Read the model definition and answer for the solid it produces. Units are mm, in the model's axes. Coordinates: 2 decimals unless noted, no trailing zeros. Loops run counter-clockwise (first coordinate to the right, second up) from the corner with the lowest first, then second, coordinate; pieces in that order, holes last. Notation, with made-up numbers: (35, 75) - (79, 75) arc R22 ccw to (79, 104) - close; hole circle Ø9 at (47, 0.25). An arc over 180 degrees is marked (long way). Use one line per item in the form item = value. Start each with the question number.
1) A cutting plane is placed at B-B (y = -42). Give the vertices of the cut face in (x, z), and give its area (3 significant figures).
2) Each of these flat-tipped pins is pushed along its axis until it touches: P1, Ø5, axis at x = 71.51, y = -164.45, coming from the +Z side; P2, Ø0.9, axis at x = 37, z = -2.5, coming from the +Y side. Where does it stop, or does it pass through?
3) Consider line 1 (X direction, y = -184, z = -2.6); line 2 (X direction, y = -74.45, z = -1.95); line 3 (Y direction, x = 67, z = -1.8). Determine where each line is inside the solid, lowest interval first.
4) A cutting plane is placed at A-A (y = -184). Give the vertices of the cut face in (x, z).
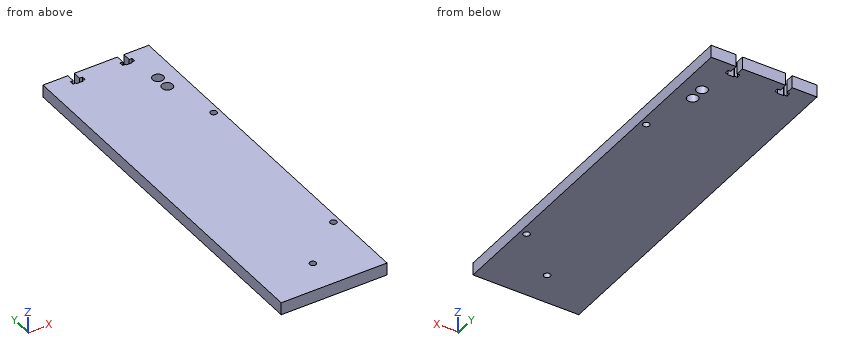
from build123d import *

# Parameters (mm, degrees)
SZKIC1_W                    = 51
SZKIC1_H                    = 179
DODANIE_WYCI_GNI_CIE1_DEPTH = 6
SZKIC3_R                    = 1.55
WYTNIJ_WYCI_GNI_CIE1_DEPTH  = 214.511356279
WYTNIJ_WYCI_GNI_CIE2_DEPTH  = 214.511356279
SZYK_LINIOWY1_COUNT         = 2
SZYK_LINIOWY1_PITCH         = 23.9
SZKIC5_R                    = 2.6
WYTNIJ_WYCI_GNI_CIE3_DEPTH  = 214.511356279
SZKIC7_R                    = 1.55
WYTNIJ_WYCI_GNI_CIE4_DEPTH  = 6


with BuildPart() as part:
    # Szkic1 → Dodanie-wyciągnięcie1 (new body)
    with BuildSketch(Plane.XY):
        with Locations((49.005699514, -110.5)):
            Rectangle(SZKIC1_W, SZKIC1_H)
    extrude(amount=-DODANIE_WYCI_GNI_CIE1_DEPTH)

    # Szkic3 → Wytnij-wyciągnięcie1 (cut, through all)
    with BuildSketch(Plane(origin=(0, 0, -6), x_dir=(-1, 0, 0), z_dir=(0, 0, -1))):
        with Locations((-71.505699514, -164.45)):
            Circle(SZKIC3_R)
        with Locations((-71.505699514, -74.45)):
            Circle(SZKIC3_R)
    extrude(amount=-WYTNIJ_WYCI_GNI_CIE1_DEPTH, mode=Mode.SUBTRACT)

    # Szkic4 → Wytnij-wyciągnięcie2 (cut, through all)
    with BuildSketch(Plane(origin=(0, 0, -6), x_dir=(-1, 0, 0), z_dir=(0, 0, -1))):
        Polygon((-59.405699514, -21), (-62.505699514, -21), (-62.505699514, -25), (-63.880699514, -25), (-63.880699514, -27), (-62.505699514, -27), (-62.505699514, -27.5), (-59.405699514, -27.5), (-59.405699514, -27), (-58.030699514, -27), (-58.030699514, -25), (-59.405699514, -25), align=None)
    wytnij_wyci_gni_cie2 = extrude(amount=-WYTNIJ_WYCI_GNI_CIE2_DEPTH, mode=Mode.SUBTRACT)

    # Szyk liniowy1: Wytnij-wyciągnięcie2 ×2
    with Locations(*[(-i * SZYK_LINIOWY1_PITCH, 0, 0) for i in range(1, SZYK_LINIOWY1_COUNT)]):
        add(wytnij_wyci_gni_cie2, mode=Mode.SUBTRACT)

    # Szkic5 → Wytnij-wyciągnięcie3 (cut, through all)
    with BuildSketch(Plane(origin=(0, 0, -6), x_dir=(-1, 0, 0), z_dir=(0, 0, -1))):
        with Locations((-65.505699514, -42)):
            Circle(SZKIC5_R)
        with Locations((-65.505699514, -49)):
            Circle(SZKIC5_R)
    extrude(amount=-WYTNIJ_WYCI_GNI_CIE3_DEPTH, mode=Mode.SUBTRACT)

    # Szkic7 → Wytnij-wyciągnięcie4 (cut)
    with BuildSketch(Plane(origin=(0, 0, -6), x_dir=(-1, 0, 0), z_dir=(0, 0, -1))):
        with Locations((-49.055699514, -184)):
            Circle(SZKIC7_R)
    extrude(amount=-WYTNIJ_WYCI_GNI_CIE4_DEPTH, mode=Mode.SUBTRACT)


solid = part.part
Found:
q1.outline = (23.51, -6) - (62.91, -6) - (62.91, 0) - (23.51, 0) - close; (68.11, -6) - (74.51, -6) - (74.51, 0) - (68.11, 0) - close
q1.area = 275 mm^2
q2.P1 = 0
q2.P2 = -27.5
q3.line_1 = 23.51 to 47.51, 50.61 to 74.51
q3.line_2 = 23.51 to 69.96, 73.06 to 74.51
q3.line_3 = -200 to -51.13, -46.87 to -44.13, -39.87 to -21
q4.outline = (23.51, -6) - (47.51, -6) - (47.51, 0) - (23.51, 0) - close; (50.61, -6) - (74.51, -6) - (74.51, 0) - (50.61, 0) - close
